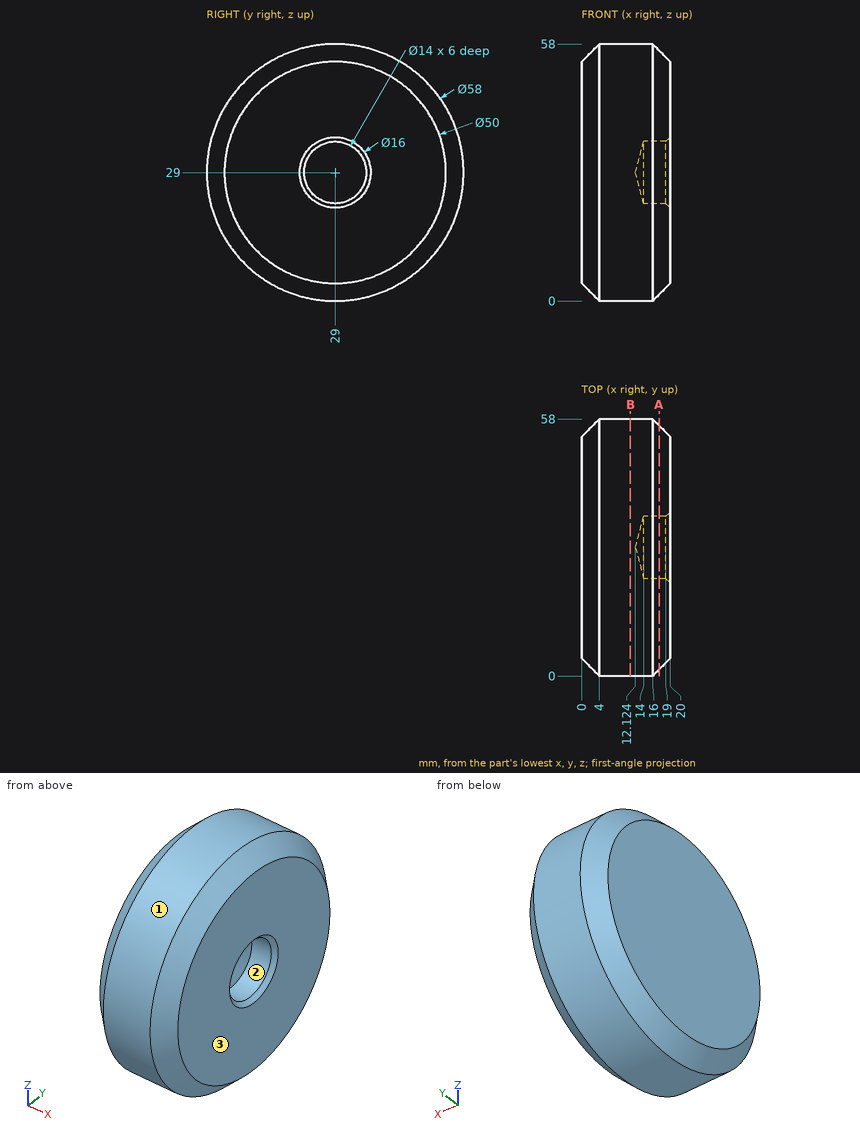
Answer from the drawing. Dimensions are ordinates in mm from the lowest x, y and z of the part. Give positions to 0.01 mm unless a question says otherwise; leave off trailing zeros. Write each loop counter-clockwise with the first axis right and the second up, starting at its lowest first coordinate (ties: lowest second). Pieces come first, ordered by that corner, then holes. Notation, with made-up numbers: (49.25, 42) -> (65.25, 42) arc R31 ccw to (65.25, 75) -> close; hole circle Ø10 at (84, -20.5). An arc over 180 degrees is marked (long way). Use a Markdown table: item, result.
(1) Determine the mould class of the marked faces 1, 2 and 3 for opening direction Z: released by +Z, released by -Z, zero draft, split by the parting line, or undercut.
Return value:
| item | result |
|---|---|
| face 1 | split by the parting line |
| face 2 | undercut |
| face 3 | zero draft |
(2) Find the intervals of material crossed by probe 1 along Z at (x, y) = (15.1, 29); probe 2 along Z at (x, y) = (17.35, 29); probe 3 along Y at (x, z) = (16.3, 29), in increasing order. Write a range as from..to.
Return value:
| item | result |
|---|---|
| probe 1 | 0..22, 36..58 |
| probe 2 | 1.35..22, 36..56.65 |
| probe 3 | 0.3..22, 36..57.7 |
(3) Flat-ended cylindrical pins translate along their axes: P1, Ø8, axis at x = 17.5, y = 40, coming from the +Z side; P2, Ø3, axis at x = 15.5, z = 50.5, coming from the +Y side; P3, Ø4, axis at x = 8.5, z = 21.5, coming from the -Y side. Find the tip coordinate at first contact, or state that the pin passes through.
Return value:
| item | result |
|---|---|
| P1 | z = 57.07 |
| P2 | y = 50 |
| P3 | y = 0.53 |
(4) Section A-A, the plane x = 17.5 is taken. Determine the outline of the cut face in (y, z), then the cut area to 3 significant figures.
Return value:
| item | result |
|---|---|
| outline | circle Ø55 at (29, 29); hole circle Ø14 at (29, 29) |
| area | 2,220 mm2 |
(5) Section B-B, the plane x = 11 is taken. Determine the outline of the cut face in (y, z).
Return value:
| item | result |
|---|---|
| outline | circle Ø58 at (29, 29) |
